Verification items for the finished model (mm, model axes). A direction names the side the tool comes from. Give positions to 0.01 mm unless a question says otherwise; leave off trailing zeros. Write each loop counter-clockwise with the first axis right and the second up, starting at its lowest first coordinate (ties: lowest second). Pieces come first, ordered by that corner, then holes. Notation, with made-up numbers: M 84.5,63 L 121.5,63 A7 cw 121.5,75 Z; hole C -26.75,-22.75 d4. An arc over 180 degrees is marked long. Answer as a JSON object with one key per item and string values.
```python
from build123d import *

# Parameters (mm, degrees)
F1_DEPTH = 25


with BuildPart() as f1:
    # F0 (on Front) → F1 (new body)
    with BuildSketch(Plane.XZ):
        Polygon((-97.923082, 42.802202), (-97.923082, 0), (-66.604404, 0), (-21.923082, 0), (-21.923082, 42.802202), (-38.208792, 61.593413), (-59.923082, 61.593413), (-81.637373, 61.593413), align=None)
        Polygon((-21.923082, 42.802202), (-21.923082, 0), (9.395596, 0), (54.076918, 0), (54.076918, 42.802202), (37.791208, 61.593413), (16.076918, 61.593413), (-5.637373, 61.593413), align=None)
        Polygon((54.076918, 42.802202), (54.076918, 0), (130.076918, 0), (130.076918, 42.802202), (113.791208, 61.593413), (92.076918, 61.593413), (70.362627, 61.593413), align=None)
    extrude(amount=F1_DEPTH)


solid = f1.part
```
1) Section check D-D on x = -14.5. Record the boundary of the cut face in (y, z).
Completed:
{"outline": "M -25,0 L 0,0 L 0,51.37 L -25,51.37 Z"}
2) Access from +Z, -Z, +X, -X, +Y, -Y to the whole of each face (thin tool, end or side, straight path). Record for faces 1 (the face through (122.048, -12.325, 52.066)), 2 (the face through (62.334, -12.325, 52.329)).
Completed:
{"face 1": "+Z, +X, +Y, -Y", "face 2": "+Z, +Y, -Y"}
3) Section check A-A on z = 57. Record the boundary of the cut face in (x, y).
Completed:
{"outline": "M -85.62,-25 L -34.23,-25 L -34.23,0 L -85.62,0 Z; M -9.62,-25 L 41.77,-25 L 41.77,0 L -9.62,0 Z; M 66.38,-25 L 117.77,-25 L 117.77,0 L 66.38,0 Z"}
4) Release check for a two-part mould opening along X. For faces 3 (the face through (-89.666, -12.325, 52.329)), 4 (the face through (14, 0, 31)), 5 (the face through (46.048, -12.325, 52.066)) record: pulls with the +X half, pulls with the -X half, needs draft (parallel to the pull), parting line crosses it, or undercut.
Completed:
{"face 3": "pulls with the -X half", "face 4": "needs draft", "face 5": "undercut"}
5) Section check C-C on x = 67. Record the boundary of the cut face in (y, z), and give its area (3 significant figures).
Completed:
{"outline": "M -25,0 L 0,0 L 0,57.71 L -25,57.71 Z", "area": "1,440 mm2"}
6) Section check B-B on y = -16. Record the boundary of the cut face in (x, z).
Completed:
{"outline": "M -97.92,0 L 130.08,0 L 130.08,42.8 L 113.79,61.59 L 70.36,61.59 L 54.08,42.8 L 37.79,61.59 L -5.64,61.59 L -21.92,42.8 L -38.21,61.59 L -81.64,61.59 L -97.92,42.8 Z"}
7) Thickness scan on L1, parallel to X at y = -18, z = 55.5; L2, parallel to X at y = -5.5, z = 46.5; L3, parallel to Z at x = 119, y = -6.75. Record the ranges inside material, lowest first.
Completed:
{"L1": "x = -86.92 to -32.93, -10.92 to 43.07, 65.08 to 119.07", "L2": "x = -94.72 to -25.13, -18.72 to 50.87, 57.28 to 126.87", "L3": "z = 0 to 55.58"}
